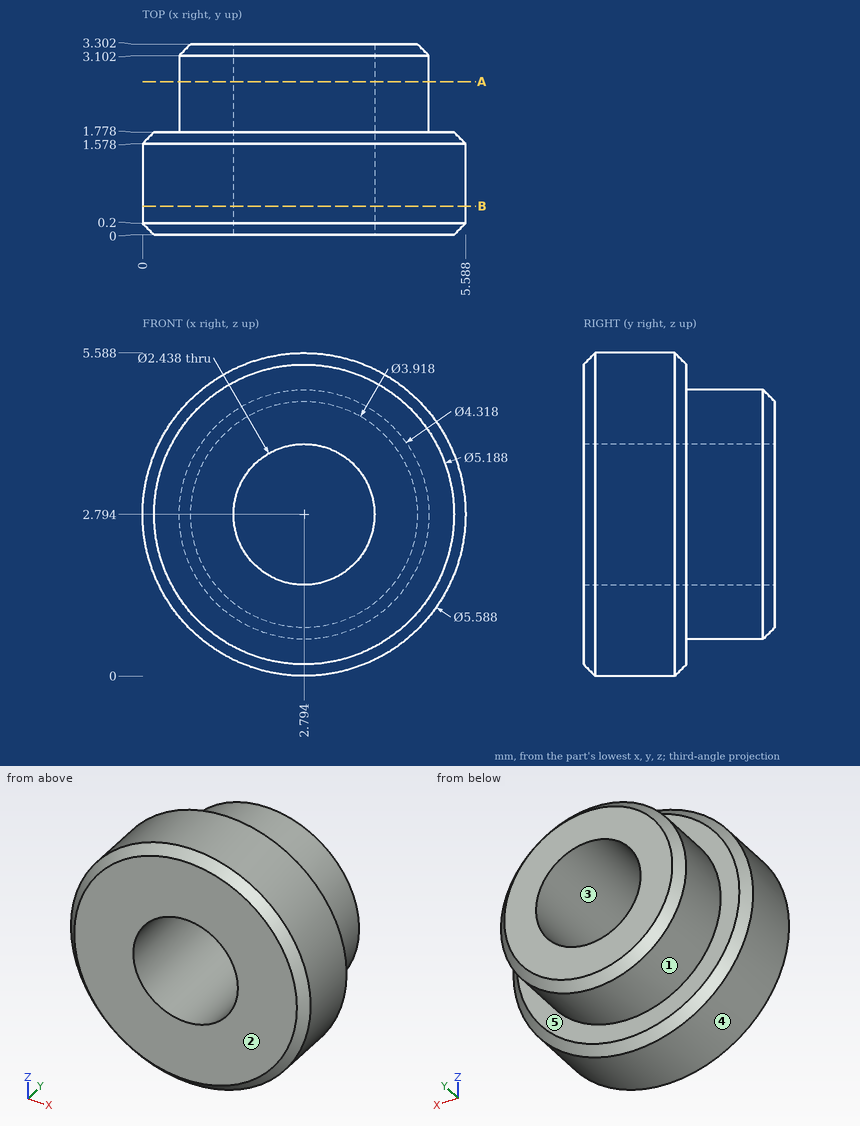
Input: dimensioned drawing with shaded views. Units: mm. Origin: part minimum x, y, z. A direction names the side the tool comes from. Round coordinates to 2 decimals unless told otherwise and drop trailing zeros. Order: outer loops, then holes, each group sorted by start corner. A loop starts at its lowest first (then second) coordinate and runs counter-clockwise, first axis right, second up. Notation, with made-up numbers: (-32, 75.5) - (-13, 75.5) arc R31 ccw to (-13, 103.5) - close; hole circle Ø1 at (-13, 57.5). An arc over 180 degrees is marked (long way). Write item = value, one per line. Start each with the question number.
Q1. Ray query, line 1 (X direction, y = 2.8, z = 2.8) (1 decimal); line 2 (Y direction, x = 0.85, z = 3.95). Return the intervals inside material, ascending. Write a range as from..to.
Q2. Pull-direction query (X, two-part tool) for the marked faces 3, 4 and 5; classes: +X half, -X half, draft (parallel to the pull), parting line (faces both ways), or undercut.
Q3. Cut plane B-B on y = 0.5. Return the cut outline in (x, z).
Q4. Pin query (flat end, axial travel): pin 1 (2.5 mm diameter, centred on x = 3.5, z = 3.5, fed in from +Y); pin 2 (1 mm diameter, centred on x = 4.5, y = 2.5, fed in from +Z) (1 decimal); pin 3 (1.5 mm diameter, centred on y = 1, z = 1, fed in from +X) (1 decimal). Return the tip coordinate at first contact, or that it passes through.
Q5. Cut plane A-A on y = 2.65. Return the cut outline in (x, z).
Q6. Access query for the marked faces 1 and 2. Directions: +Z, -Z, +X, -X, +Y, -Y. A direction counts if a zero-diameter tool reaches every point of the face in a straight line with its end or side. Return the directions, or none.
Outcome:
q1.line_1 = 0.6..1.6, 4..5
q1.line_2 = 0..1.78
q2.face_3 = undercut
q2.face_4 = parting line
q2.face_5 = draft
q3.outline = circle Ø5.59 at (2.79, 2.79); hole circle Ø2.44 at (2.79, 2.79)
q4.pin_1 = 3.3
q4.pin_2 = 4.6
q4.pin_3 = 5.4
q5.outline = circle Ø4.32 at (2.79, 2.79); hole circle Ø2.44 at (2.79, 2.79)
q6.face_1 = +Y
q6.face_2 = +Z, -Z, +X, -X, -Y
